Autodesk Inventor part; units mm, degrees
ref_plane "YZ Plane" through (0, 0, 0) normal (1, 0, 0) x (0, 1, 0)
ref_plane "XZ Plane" through (0, 0, 0) normal (0, 1, 0) x (-1, 0, 0)
ref_plane "XY Plane" through (0, 0, 0) normal (0, 0, 1) x (1, 0, 0)
sketch "Sketch1" plane through (0, 0, 0) normal (0, 1, 0) x (-1, 0, 0)
  circle A0 centre (0, 0) radius 2.4892
  circle A1 centre (0, -22.225) radius 3.2512
  circle A2 centre (0, -44.45) radius 3.2512
  circle A3 centre (-22.225, 0) radius 3.2512
  circle A4 centre (-44.45, 0) radius 3.2512
  line L0 (12.7, 12.7) -> (-57.15, 12.7)
  line L1 (-57.15, 12.7) -> (-57.15, -12.7)
  line L2 (-57.15, -12.7) -> (-12.7, -12.7)
  line L3 (-12.7, -12.7) -> (-12.7, -57.15)
  line L4 (-12.7, -57.15) -> (12.7, -57.15)
  line L5 (12.7, -57.15) -> (12.7, 12.7)
  dimension "d0" = 4.9784
  dimension "d1" = 6.5024
  dimension "d2" = 22.225
  dimension "d3" = 22.225
  dimension "d4" = 22.225
  dimension "d5" = 22.225
  dimension "d6" = 12.7
  dimension "d7" = 12.7
  dimension "d8" = 12.7
  dimension "d9" = 12.7
  dimension "d10" = 12.7
  dimension "d11" = 12.7
extrude "Extrusion1" add sketch "Sketch1" along normal blind 4.7625
fillet "Fillet1" radius 19.05 1 edges at (12.7, 2.3813, -12.7)
fillet "Fillet2" radius 4.7625 5 edges at (57.15, 2.3813, -12.7) (57.15, 2.3813, 12.7) (12.7, 2.3813, -57.15) (-12.7, 2.3813, -57.15) (-12.7, 2.3813, 12.7)
properties part number "STRU_016_FrameBracket2_90" material "Aluminum 6061"
CAD build for the part. Positions are in the model's coordinates, mm. A direction names the side the tool comes from. Give positions to 0.01 mm unless a question says otherwise; leave off trailing zeros. Write each loop counter-clockwise with the first axis right and the second up, starting at its lowest first coordinate (ties: lowest second). Pieces come first, ordered by that corner, then holes. Notation, with made-up numbers: M 69.25,38.25 L 128.25,38.25 A23 ccw 128.25,57.25 Z; hole C 53,-15 d9. An arc over 180 degrees is marked long. Put each result on its own line as item: value. Start each with the question number.
(1) Band-saw the part on A-A, the plane x = 44.45. Write the cut outline in (y, z), and give its area (3 significant figures).
(2) Band-saw the part on C-C, the plane z = 0. Write the cut outline in (x, y), and give its area (3 significant figures).
(3) Which spindle directions (+Z, -Z, +X, -X, +Y, -Y) get a long thin tool onto all of the face, cutting with end or side? Do faces 1 (the face through (12.7, 2, -42)), 2 (the face through (2.396, 2.348, -46.647)). Say none if no direction does.
(4) Mould opens along Z. For faces 3 (the face through (55.79, 2.41, -11.27)), 4 (the face through (0.42, 2.35, -25.45)), 5 (the face through (57.15, 2, 0)), 6 (the face through (55.72, 2.41, 11.34)) say: +Z half, -Z half, draft (parallel to the pull), parting line (faces both ways), or undercut.
(5) Probe L1, parallel to Z at x = 0, y = 1.7; L2, parallel to Z at x = -0.5, y = 4.35; L3, parallel to Z at x = 44.45, y = 1.3. List the from-to ranges inside material, lowest first.
(6) Flat gauge pins, fed straight in: pin 1 Ø3 at (x, z) = (0, 0) entering from -Y; pin 2 Ø1.5 at (y, z) = (3.5, -28) entering from +X; pin 3 Ø2.5 at (y, z) = (1.5, -45) entering from +X; pin 4 Ø2.5 at (x, y) = (40, 2) entering from -Z. Where does each tip first touch, or does it go through?
(7) Band-saw the part on B-B, the plane x = 0. Write the cut outline in (y, z), and give its area (3 significant figures).
(8) Band-saw the part on D-D, the plane z = -44.45. Write the cut outline in (x, y), and give its area (3 significant figures).
Response values:
1. outline: M 0,-12.7 L 4.76,-12.7 L 4.76,-3.25 L 0,-3.25 Z; M 0,3.25 L 4.76,3.25 L 4.76,12.7 L 0,12.7 Z
1. area: 90.0 mm2
2. outline: M -12.7,0 L -2.49,0 L -2.49,4.76 L -12.7,4.76 Z; M 2.49,0 L 18.97,0 L 18.97,4.76 L 2.49,4.76 Z; M 25.48,0 L 41.2,0 L 41.2,4.76 L 25.48,4.76 Z; M 47.7,0 L 57.15,0 L 57.15,4.76 L 47.7,4.76 Z
2. area: 247 mm2
3. face 1: -Z, +X, +Y, -Y
3. face 2: +Y, -Y
4. face 3: -Z half
4. face 4: undercut
4. face 5: draft
4. face 6: +Z half
5. L1: z = -57.15 to -47.7, -41.2 to -25.48, -18.97 to -2.49, 2.49 to 12.7
5. L2: z = -57.15 to -47.66, -41.24 to -25.44, -19.01 to -2.44, 2.44 to 12.7
5. L3: z = -12.7 to -3.25, 3.25 to 12.7
6. pin 1: passes through
6. pin 2: stops at x = 13.24
6. pin 3: stops at x = 12.7
6. pin 4: stops at z = -12.7
7. outline: M 0,-57.15 L 4.76,-57.15 L 4.76,-47.7 L 0,-47.7 Z; M 0,-41.2 L 4.76,-41.2 L 4.76,-25.48 L 0,-25.48 Z; M 0,-18.97 L 4.76,-18.97 L 4.76,-2.49 L 0,-2.49 Z; M 0,2.49 L 4.76,2.49 L 4.76,12.7 L 0,12.7 Z
7. area: 247 mm2
8. outline: M -12.7,0 L -3.25,0 L -3.25,4.76 L -12.7,4.76 Z; M 3.25,0 L 12.7,0 L 12.7,4.76 L 3.25,4.76 Z
8. area: 90.0 mm2
